Autodesk Inventor part; units mm, degrees
ref_plane "Work Plane1" through (0, 0, 0) normal (0, 0, 1) x (1, 0, 0)
ref_plane "YZ Plane" through (0, 0, 0) normal (1, 0, 0) x (0, 1, 0)
ref_plane "XZ Plane" through (0, 0, 0) normal (0, 1, 0) x (-1, 0, 0)
ref_plane "Work Plane1" through (0, 0, 0) normal (0, 0, 1) x (1, 0, 0)
sketch "Sketch1" plane through (0, 0, 0) normal (0, 0, 1) x (1, 0, 0)
  line L0 (-66.675, -19.05) -> (66.675, -19.05)
  line L1 (66.675, -19.05) -> (66.675, 19.05)
  line L2 (66.675, 19.05) -> (-66.675, 19.05)
  line L3 (-66.675, 19.05) -> (-66.675, -19.05)
  circle A0 centre (61.0954, -13.4704) radius 1.778 construction
  circle A1 centre (59.7602, -6.9148) radius 1.778 construction
  circle A2 centre (57.15, 0) radius 2.032 construction
  circle A3 centre (54.5398, -6.9148) radius 1.778 construction
  circle A4 centre (53.2046, -13.4704) radius 1.778 construction
  circle A5 centre (54.5398, 6.9148) radius 1.778 construction
  circle A6 centre (53.2046, 13.4704) radius 1.778 construction
  circle A7 centre (59.7602, 6.9148) radius 1.778 construction
  circle A8 centre (61.0954, 13.4704) radius 1.778 construction
  circle A9 centre (47.625, 9.779) radius 1.778 construction
  circle A10 centre (47.625, -9.779) radius 1.778 construction
  circle A11 centre (34.1546, -13.4704) radius 1.778 construction
  circle A12 centre (42.0454, -13.4704) radius 1.778 construction
  circle A13 centre (40.7102, -6.9148) radius 1.778 construction
  circle A14 centre (38.1, 0) radius 2.032 construction
  circle A15 centre (40.7102, 6.9148) radius 1.778 construction
  circle A16 centre (42.0454, 13.4704) radius 1.778 construction
  circle A17 centre (35.4898, 6.9148) radius 1.778 construction
  circle A18 centre (34.1546, 13.4704) radius 1.778 construction
  circle A19 centre (35.4898, -6.9148) radius 1.778 construction
  circle A20 centre (34.1546, -13.4704) radius 1.778 construction
  circle A21 centre (28.575, -9.779) radius 1.778 construction
  circle A22 centre (28.575, 9.779) radius 1.778 construction
  circle A23 centre (21.6602, 6.9148) radius 1.778 construction
  circle A24 centre (16.4398, 6.9148) radius 1.778 construction
  circle A25 centre (15.1046, 13.4704) radius 1.778 construction
  circle A26 centre (22.9954, 13.4704) radius 1.778 construction
  circle A27 centre (19.05, 0) radius 2.032 construction
  circle A28 centre (21.6602, -6.9148) radius 1.778 construction
  circle A29 centre (22.9954, -13.4704) radius 1.778 construction
  circle A30 centre (15.1046, -13.4704) radius 1.778 construction
  circle A31 centre (16.4398, -6.9148) radius 1.778 construction
  circle A32 centre (9.525, -9.779) radius 1.778 construction
  circle A33 centre (9.525, 9.779) radius 1.778 construction
  circle A34 centre (3.9454, 13.4704) radius 1.778 construction
  circle A35 centre (2.6102, 6.9148) radius 1.778 construction
  circle A36 centre (-2.6102, 6.9148) radius 1.778 construction
  circle A37 centre (-3.9454, 13.4704) radius 1.778 construction
  circle A38 centre (0, 0) radius 2.032 construction
  circle A39 centre (-2.6102, -6.9148) radius 1.778 construction
  circle A40 centre (2.6102, -6.9148) radius 1.778 construction
  circle A41 centre (3.9454, -13.4704) radius 1.778 construction
  circle A42 centre (-3.9454, -13.4704) radius 1.778 construction
  circle A43 centre (-9.525, -9.779) radius 1.778 construction
  circle A44 centre (-9.525, 9.779) radius 1.778 construction
  circle A45 centre (-15.1046, 13.4704) radius 1.778 construction
  circle A46 centre (-22.9954, 13.4704) radius 1.778 construction
  circle A47 centre (-21.6602, 6.9148) radius 1.778 construction
  circle A48 centre (-16.4398, 6.9148) radius 1.778 construction
  circle A49 centre (-19.05, 0) radius 2.032 construction
  circle A50 centre (-21.6602, -6.9148) radius 1.778 construction
  circle A51 centre (-16.4398, -6.9148) radius 1.778 construction
  circle A52 centre (-15.1046, -13.4704) radius 1.778 construction
  circle A53 centre (-22.9954, -13.4704) radius 1.778 construction
  circle A54 centre (-28.575, -9.779) radius 1.778 construction
  circle A55 centre (-28.575, 9.779) radius 1.778 construction
  circle A56 centre (-34.1546, 13.4704) radius 1.778 construction
  circle A57 centre (-42.0454, 13.4704) radius 1.778 construction
  circle A58 centre (-40.7102, 6.9148) radius 1.778 construction
  circle A59 centre (-35.4898, 6.9148) radius 1.778 construction
  circle A60 centre (-38.1, 0) radius 2.032 construction
  circle A61 centre (-35.4898, -6.9148) radius 1.778 construction
  circle A62 centre (-40.7102, -6.9148) radius 1.778 construction
  circle A63 centre (-34.1546, -13.4704) radius 1.778 construction
  circle A64 centre (-42.0454, -13.4704) radius 1.778 construction
  circle A65 centre (-47.625, -9.779) radius 1.778 construction
  circle A66 centre (-53.2046, -13.4704) radius 1.778 construction
  circle A67 centre (-54.5398, -6.9148) radius 1.778 construction
  circle A68 centre (-57.15, 0) radius 2.032 construction
  circle A69 centre (-59.7602, -6.9148) radius 1.778 construction
  circle A70 centre (-61.0954, -13.4704) radius 1.778 construction
  circle A71 centre (-59.7602, 6.9148) radius 1.778 construction
  circle A72 centre (-54.5398, 6.9148) radius 1.778 construction
  circle A73 centre (-53.2046, 13.4704) radius 1.778 construction
  circle A74 centre (-61.0954, 13.4704) radius 1.778 construction
extrude "Extrusion2" add sketch "Sketch1" along normal blind 5.08
sketch "Sketch2" plane through (0, 0, 5.08) normal (0, 0, 1) x (1, 0, 0)
  circle A0 centre (-53.2046, -13.4704) radius 1.9685 construction
  circle A1 centre (-53.2046, -13.4704) radius 2.8702 construction
  circle A2 centre (-42.0454, -13.4704) radius 1.9685 construction
  circle A3 centre (-42.0454, -13.4704) radius 2.8702 construction
  point P0 (0, 0)
  dimension "d37" = 5.7404
  dimension "d38" = 5.7404
ref_plane "Work Plane2" through (-43.561, -19.05, 0) normal (-1, 0, 0) x (0, 0, 1)
sketch "Sketch3" plane through (-43.561, -19.05, 0) normal (-1, 0, 0) x (0, 0, 1)
  line L0 (0, 6.35) -> (5.08, 6.35) construction
  line L1 (5.08, 0) -> (5.08, 38.1)
  line L2 (0, 0) -> (5.08, 0)
  line L3 (0, 0) -> (0, 38.1)
  line L4 (0, 31.75) -> (5.08, 31.75) construction
  line L5 (0, 38.1) -> (5.08, 38.1)
  line L6 (8.89, 31.75) -> (8.89, 6.35) construction
  circle A0 centre (24.765, 19.05) radius 15.875
  circle A1 centre (24.765, 19.05) radius 1.9685
  line L7 (24.765, 19.05) -> (34.925, 19.05) construction
  line L8 (24.765, 34.925) -> (5.08, 34.925)
  line L9 (5.08, 34.925) -> (5.08, 3.175)
  line L10 (5.08, 3.175) -> (23.495, 3.175)
  arc A2 (24.765, 31.75) -> (23.495, 6.4137) centre (24.765, 19.05) ccw
  line L11 (24.765, 31.75) -> (24.765, 34.925)
  line L12 (23.495, 3.175) -> (23.495, 6.4137)
  line L13 (24.765, 17.0815) -> (24.765, 21.0185)
  line L14 (5.08, 21.0185) -> (5.08, 17.0815)
  line L15 (5.08, 19.05) -> (5.08, 29.21)
  line L16 (5.08, 19.05) -> (5.08, 8.89)
  circle A3 centre (14.605, 19.05) radius 1.9685
  point P0 (0, 19.05)
  dimension "d45" = 31.75
  dimension "d40" = 6.35
  dimension "d41" = 6.35
  dimension "d43" = 15.875
  dimension "d46" = 3.937
  dimension "d51" = 3.81
  dimension "d52" = 19.05
  dimension "d61" = 25.4
  dimension "d62" = 10.16
  dimension "d63" = 10.16
  dimension "d66" = 10.16
  dimension "d67" = 3.937
ref_plane "Work Plane3" through (0, -19.05, 0) normal (1, 0, 0) x (0, 0, -1)
extrude "Extrusion4" add sketch "Sketch3" along normal blind 1.905 and the other way blind 1.905 contours L1 L8 A0 L12 L10 | L12 A2 L11 A0 | A0 L11 A2 L12
mirror "Mirror2" about plane through (0, -19.05, 0) normal (1, 0, 0) of "Extrusion4"
fillet "Fillet3" radius 3.175 8 edges at (-41.656, 0, 5.08) (-43.561, -15.875, 5.08) (-45.466, 0, 5.08) (-43.561, 15.875, 5.08) (41.656, 0, 5.08) (43.561, 15.875, 5.08) (45.466, 0, 5.08) (43.561, -15.875, 5.08)
ref_plane "Work Plane4" through (-66.675, 0, 0) normal (0, 1, 0) x (1, 0, 0)
sketch "Sketch5" plane through (0, 0, 0) normal (0, 0, -1) x (-1, 0, 0)
  line L0 (66.675, 19.05) -> (66.675, -19.05)
  line L1 (-66.675, 19.05) -> (66.675, 19.05)
  line L2 (66.675, -19.05) -> (-66.675, -19.05)
  point P0 (0, 0)
  point P1 (62.9666, 13.97)
  point P2 (62.9666, -13.97)
  dimension "d73" = 3.7084
  dimension "d74" = 3.7084
  dimension "d75" = 5.08
  dimension "d76" = 5.08
hole "Hole1" at (-62.9666, -13.97, 0) at (-62.9666, 13.97, 0) direction (0, 0, 1) diameter 3.937 end through all
sketch "Sketch6" plane through (0, 0, 5.08) normal (0, 0, 1) x (1, 0, 0)
  line L0 (15.875, 12.7) -> (-34.925, 12.7)
  line L1 (-34.925, 12.7) -> (-34.925, -12.7)
  line L2 (-34.925, -12.7) -> (15.875, -12.7)
  line L3 (15.875, -12.7) -> (15.875, 12.7)
  line L4 (-38.481, -19.05) -> (38.481, -19.05)
  line L5 (38.481, 19.05) -> (-38.481, 19.05)
  line L6 (-66.675, 19.05) -> (-66.675, -19.05)
  line L7 (66.675, -19.05) -> (66.675, 19.05)
  line L8 (23.7236, -12.7) -> (38.481, -12.7)
  line L9 (38.481, 12.7) -> (23.7236, 12.7)
  line L10 (23.7236, 12.7) -> (23.7236, -12.7)
  line L11 (38.481, 19.05) -> (38.481, -19.05)
  line L12 (38.481, -12.7) -> (38.481, 12.7)
  point P0 (0, 0)
  dimension "d84" = 6.35
  dimension "d85" = 6.35
  dimension "d86" = 31.75
  dimension "d87" = 50.8
  dimension "d102" = 42.9514
extrude "Extrusion5" cut sketch "Sketch6" against normal through all
fillet "Fillet4" radius 3.175 4 edges at (15.875, -12.7, 2.54) (-34.925, -12.7, 2.54) (-34.925, 12.7, 2.54) (15.875, 12.7, 2.54)
sketch "Sketch7" plane through (0, 0, 0) normal (0, 0, -1) x (-1, 0, 0)
  line L0 (-66.675, -19.05) -> (-66.675, 19.05)
  line L1 (66.675, -19.05) -> (-66.675, -19.05)
  line L2 (-66.675, 19.05) -> (66.675, 19.05)
  point P0 (0, 0)
  point P1 (-20.0406, 13.97)
  point P2 (-20.0406, -13.97)
  dimension "d91" = 46.6344
  dimension "d92" = 46.6344
  dimension "d93" = 5.08
  dimension "d94" = 5.08
hole "Hole2" at (20.0406, 13.97, 0) at (20.0406, -13.97, 0) direction (0, 0, 1) diameter 3.937 end through all
fillet "Fillet5" radius 3.175 4 edges at (38.481, 12.7, 2.54) (23.7236, 12.7, 2.54) (38.481, -12.7, 2.54) (23.7236, -12.7, 2.54)
properties part number "phone mount pivot"
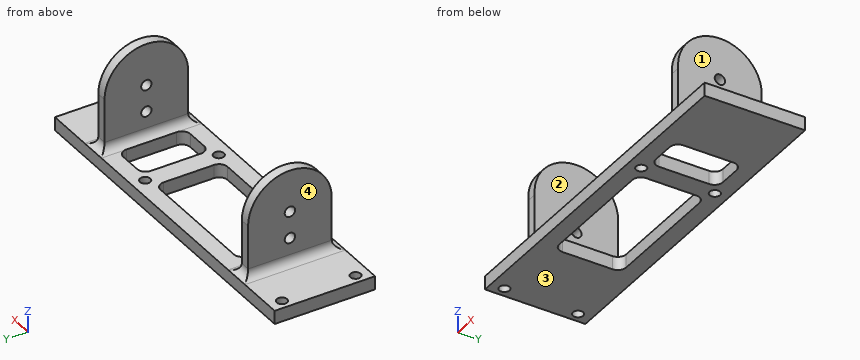
For this review, take the finished solid that the model builds, in its own axes (mm). Face numbers are marked on the shaded views. A direction names the side the tool comes from. Give positions to 0.01 mm unless a question says otherwise; leave off trailing zeros. Loops run counter-clockwise (first coordinate to the right, second up) from the corner with the lowest first, then second, coordinate; pieces in that order, holes last.
Item 1: Take a section at A-A, the plane x = 1. State the section outline as (y, z) points.
Item 2: Tool access review of the marked faces 1, 2, 3 and 4: name each direction out of +Z, -Z, +X, -X, +Y, -Y from which nothing blocks a thin tool from reaching the whole face with its end or side.
Item 3: Insertion check: pin 1 (4.5 mm diameter, centred on x = 20.04, y = 13.97, fed in from +Z); pin 2 (12 mm diameter, centred on y = -9.5, z = 25, fed in from -X); pin 3 (16 mm diameter, centred on y = -3.5, z = 31, fed in from +X); pin 4 (3 mm diameter, centred on x = 20.04, y = -13.97, fed in from -Z). Each pin has a flat end and moves straight along its axis. Give the tip position at first contact, or say it passes through.
Item 4: For line 1 along X through (y, z) = (-13.97, 1.6) (3 decimals); line 2 along X through (y, z) = (15.5, 15); line 3 along Y through (x, z) = (4, 5), list the stretches that pass through material, from the lowest coordinate up.
Item 5: Take a section at C-C, the plane y = 13.97. State the section outline as (x, z) points (1 decimal).
Item 6: Take a section at B-B, the plane x = -43. Give the number of separate pieces and of enclosed holes in the cut face, and give its area (3 significant figures).
Item 7: Take a section at D-D, the plane z = 32.5. State the section outline as (x, y) points.
Calculated:
1. outline: (-19.05, 0) - (-12.7, 0) - (-12.7, 5.08) - (-19.05, 5.08) - close; (12.7, 0) - (19.05, 0) - (19.05, 5.08) - (12.7, 5.08) - close
2. face 1: +Z, +X, +Y, -Y
2. face 2: +Z, +Y, -Y
2. face 3: -Z, +X, -X, +Y, -Y
2. face 4: +Z, -X, +Y, -Y
3. pin 1: stops at z = 5.08
3. pin 2: stops at x = -45.47
3. pin 3: stops at x = 45.47
3. pin 4: passes through
4. line 1: x = -66.675 to -64.935, -60.998 to 18.072, 22.009 to 66.675
4. line 2: x = -45.47 to -41.66, 41.66 to 45.47
4. line 3: y = -19.05 to -12.7, 12.7 to 19.05
5. outline: (-66.7, 0) - (-64.9, 0) - (-64.9, 5.1) - (-66.7, 5.1) - close; (-61, 0) - (18.1, 0) - (18.1, 5.1) - (-38.5, 5.1) arc R3.2 cw to (-41.7, 8.3) - (-41.7, 32.3) - (-45.5, 32.3) - (-45.5, 8.3) arc R3.2 cw to (-48.6, 5.1) - (-61, 5.1) - close; (22, 0) - (66.7, 0) - (66.7, 5.1) - (48.6, 5.1) arc R3.2 cw to (45.5, 8.3) - (45.5, 32.3) - (41.7, 32.3) - (41.7, 8.3) arc R3.2 cw to (38.5, 5.1) - (22, 5.1) - close
6. separate pieces: 1
6. enclosed holes: 2
6. area: 1,190 mm2
7. outline: (-45.47, -13.86) - (-41.66, -13.86) - (-41.66, 13.86) - (-45.47, 13.86) - close; (41.66, -13.86) - (45.47, -13.86) - (45.47, 13.86) - (41.66, 13.86) - close
